Geometry: final body of the model. Coordinates: model frame, mm. A direction names the side the tool comes from. Coordinates: 2 decimals unless noted, no trailing zeros. Loops run counter-clockwise (first coordinate to the right, second up) from the corner with the lowest first, then second, coordinate; pieces in that order, holes last. Notation, with made-up numbers: (50.25, -29) - (86.25, -29) arc R15 ccw to (86.25, -16) - close; hole circle Ø6 at (77.5, 18). An arc over 180 degrees is marked (long way). Return JSON: item names as keys, results as strings.
from build123d import *

# Parameters (mm, degrees)
SKETCH_1_W          = 260
SKETCH_1_H          = 130
EXTRUDE_1_DEPTH     = 20
SKETCH_4_R          = 40
EXTRUDE_2_DEPTH     = 65
EXTRUDE_3_DEPTH     = 15
RIB_4_REACH         = 249.235
SKETCH_6_WALL_W     = 698.706896764
SKETCH_6_WALL_H     = 10
SKETCH_7_R          = 20
CUT_EXTRUDE_1_DEPTH = 272.661554144
FILLET_1_R          = 20


with BuildPart() as part:
    # Sketch 1 → Extrude 1 (new body)
    with BuildSketch(Plane.XY):
        Rectangle(SKETCH_1_W, SKETCH_1_H)
    extrude(amount=EXTRUDE_1_DEPTH)

    # Sketch 3 → Hole Wizard M10 _1 (revolve, cut)
    with BuildSketch(Plane(origin=(-110, 45, 20), x_dir=(0, -1, 0), z_dir=(1, 0, 0))):
        Polygon((0, 0), (0, 30.804733405), (5.5, 27.5), (5.5, 6.4), (10.7375, 6.4), (10.7375, 0.4625), (11.2, 0), align=None)
    hole_wizard_m10_1 = revolve(axis=Axis((-110, 45, 26.35), (0, 0, -1)), mode=Mode.SUBTRACT)

    # Mirror 1: Hole Wizard M10 _1 across plane
    add(hole_wizard_m10_1.mirror(Plane.ZX), mode=Mode.SUBTRACT)

    # Mirror 2: Hole Wizard M10 _1 across plane
    add(hole_wizard_m10_1.mirror(Plane(origin=(0, 0, 0), x_dir=(0, 0, 1), z_dir=(1, 0, 0))), mode=Mode.SUBTRACT)

    # Mirror 2 copy 1 sketch → Mirror 2 copy 1 (revolve, cut)
    with BuildSketch(Plane(origin=(110, -45, 20), x_dir=(0, 1, 0), z_dir=(-1, 0, 0))):
        Polygon((0, 0), (0, 30.804733405), (5.5, 27.5), (5.5, 6.4), (10.7375, 6.4), (10.7375, 0.4625), (11.2, 0), align=None)
    revolve(axis=Axis((110, -45, 26.35), (0, 0, -1)), mode=Mode.SUBTRACT)



with BuildPart() as body_2:
    # Sketch 4 → Extrude 2 (new, symmetric)
    with BuildSketch(Plane(origin=(0, 0, 0), x_dir=(1, 0, 0), z_dir=(0, 1, 0))):
        with Locations(Location((0, 160, 0), (0, 0, 270))):
            Circle(SKETCH_4_R)
    extrude(amount=EXTRUDE_2_DEPTH, both=True)


with BuildPart() as part_1:
    add(part.part)

    add(body_2.part)  # Extrude 3 merges body 2
    # Sketch 5 → Extrude 3 (add, symmetric)
    with BuildSketch(Plane(origin=(0, 0, 0), x_dir=(1, 0, 0), z_dir=(0, 1, 0))):
        with BuildLine():
            Line((-15, 122.919007565), (-15, 0))
            Line((-15, 0), (15, 0))
            Line((15, 0), (15, 122.919007565))
            ThreePointArc((15, 122.919007565), (0, 120), (-15, 122.919007565))
        make_face()
    extrude(amount=EXTRUDE_3_DEPTH, both=True)

    # Sketch 6 wall → Rib 4 (add, up to next)
    with BuildSketch(Plane(origin=(82.674351749, 0, -89.360410796), x_dir=(-0.468020539788, 0, -0.883717587432), z_dir=(-0.883717587432, 0, 0.468020539788)), mode=Mode.PRIVATE) as rib_4_sk1:
        Rectangle(SKETCH_6_WALL_W, SKETCH_6_WALL_H)
    rib_4_tool1 = extrude(rib_4_sk1.sketch, amount=RIB_4_REACH, mode=Mode.PRIVATE) - part_1.part
    rib_4 = rib_4_tool1.solids().sort_by_distance((82.674351749, 0, -89.360410796))[0]
    add(rib_4)

    # Mirror 3: Rib 4 across plane
    add(rib_4.mirror(Plane(origin=(0, 0, 0), x_dir=(0, 0, 1), z_dir=(1, 0, 0))))

    # Sketch 7 → Cut-Extrude 1 (cut, through all)
    with BuildSketch(Plane(origin=(0, 65, 0), x_dir=(1, 0, 0), z_dir=(0, 1, 0))):
        with Locations(Location((0, 160, 0), (0, 0, 270))):
            Circle(SKETCH_7_R)
    extrude(amount=-CUT_EXTRUDE_1_DEPTH, mode=Mode.SUBTRACT)

    # Fillet 1
    fillet_1_edges = [part_1.edges().sort_by_distance(p)[0] for p in [
        (-130, 65, 10),
        (130, 65, 10),
        (130, -65, 10),
        (-130, -65, 10),
    ]]
    fillet(fillet_1_edges, radius=FILLET_1_R)


solid = part_1.part
Item 1: Section query C-C, the plane z = -165. Return loops of the section in (x, y), and give its area (3 significant figures).
Worked out:
{"outline": "(-42.62, -5) - (-39.69, -5) - (-39.69, -65) - (-19.36, -65) - (-19.36, 65) - (-39.69, 65) - (-39.69, 5) - (-42.62, 5) - close; (19.36, -65) - (39.69, -65) - (39.69, -5) - (42.62, -5) - (42.62, 5) - (39.69, 5) - (39.69, 65) - (19.36, 65) - close", "area": "5,340 mm^2"}
Item 2: Ray query, probe 1 along X at (y, z) = (45, 3); probe 2 along X at (y, z) = (-45, 17.55); probe 3 along Y at (x, z) = (-110, 16). Return the intervals inside material, ascending. Write a range as from..to.
Worked out:
{"probe 1": "-130..-115.5, -104.5..104.5, 115.5..130", "probe 2": "-130..-120.74, -99.26..99.26, 120.74..130", "probe 3": "-65..-55.74, -34.26..34.26, 55.74..65"}
Item 3: Section query A-A, the plane x = 0. Return loops of the section in (y, z), and give its area (3 significant figures).
Worked out:
{"outline": "(-65, -200) - (65, -200) - (65, -180) - (-65, -180) - close; (-65, -140) - (65, -140) - (65, -120) - (15, -120) - (15, 0) - (65, 0) - (65, 20) - (-65, 20) - (-65, 0) - (-15, 0) - (-15, -120) - (-65, -120) - close", "area": "11,400 mm^2"}
Item 4: First-contact query: pin 1 Ø5 at (y, z) = (-9.5, -57) entering from +X; pin 2 Ø12 at (x, y) = (77.5, -15.5) entering from -Z; pin 3 Ø4 at (x, z) = (-13, -22.5) entering from +Y; pin 4 Ø10 at (x, y) = (110, 45) entering from -Z. Flat tips, straight axial feed; report the tip coordinate or a pass-through.
Worked out:
{"pin 1": "x = 15", "pin 2": "z = 0", "pin 3": "y = 15", "pin 4": "through"}
Item 5: Section query D-D, the plane y = 0. Return loops of the section in (x, z).
Worked out:
{"outline": "(-130, 0) - (-35.35, -178.72) arc R40 ccw to (35.35, -178.72) - (130, 0) - (130, 20) - (-130, 20) - close; hole circle Ø40 at (0, -160)"}
Item 6: Section query B-B, the plane y = 19. Return loops of the section in (x, z), and give its area (3 significant figures).
Worked out:
{"outline": "(-130, 0) - (130, 0) - (130, 20) - (-130, 20) - close; circle Ø80 at (0, -160); hole circle Ø40 at (0, -160)", "area": "8,970 mm^2"}
Item 7: Reachability of faces 1 (the face through (-60, 5, -50)), 2 (the face through (-115, 42, 13.6)), 3 (the face through (15, 10, -61)) from +Z, -Z, +X, -X, +Y, -Y: full face, straight path, thin tool, end or side. Return the list, or none.
Worked out:
{"face 1": "-X, +Y", "face 2": "+Z", "face 3": "+X, +Y"}
Item 8: Mould query, pull axis Y, two halves, no side actions, for faces 4 (the face through (100.47, -40.05, 16.61)), 5 (the face through (-2, 35, 0)), 6 (the face through (-115, -42, 13.6)), 7 (the face through (-60, -5, -50)). Classes: +Y half, -Y half, draft (parallel to the pull), parting line (faces both ways), or undercut.
Worked out:
{"face 4": "undercut", "face 5": "draft", "face 6": "undercut", "face 7": "-Y half"}
